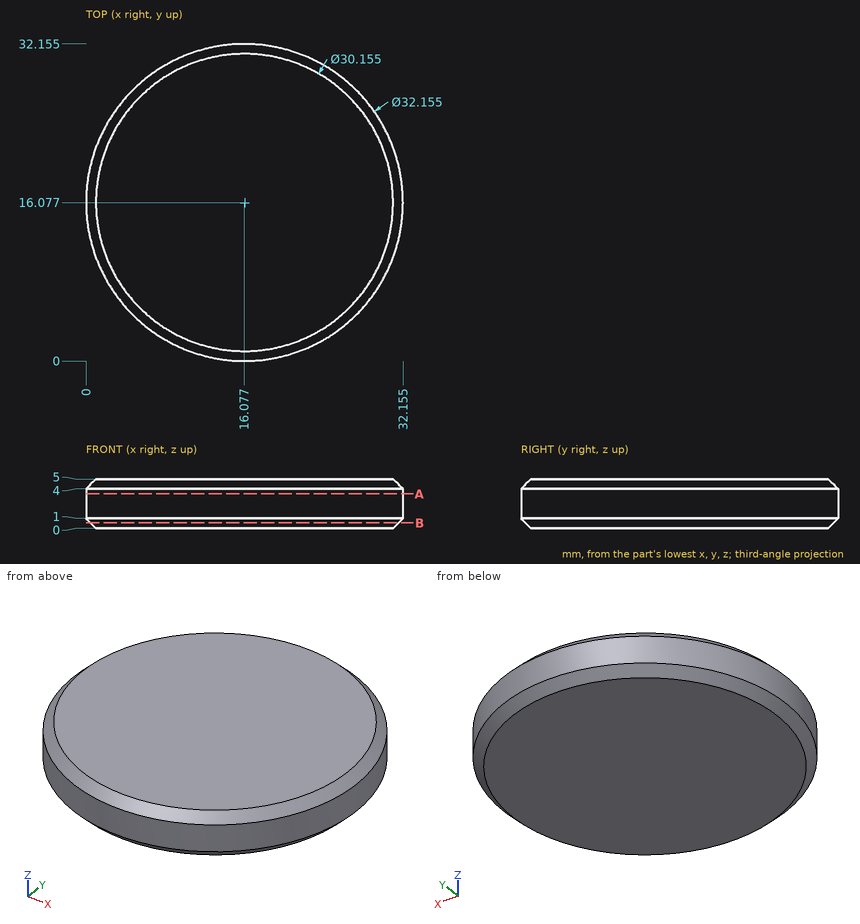
Here's the drawing with two shaded views (mm, measured from the low corner). I have some questions. Give positions to 0.01 mm unless a question says otherwise; leave off trailing zeros. Order: outer loops, then holes, each group sorted by start corner. A loop starts at its lowest first (then second) coordinate and runs counter-clockwise, first axis right, second up. Notation, with made-up numbers: (64.5, 19) -> (103.5, 19) arc R38 cw to (103.5, 57) -> close; hole circle Ø6 at (-6, 74.5). An arc over 180 degrees is marked (long way). One line per item, written item: value. Start each with the question number.
1. Imagine slicing it at A-A, the plane z = 3.5. List the corners of the cut face in (x, y) for me (1 decimal), plus the area to 3 significant figures.
2. I need wall thicknesses on probe 1 along X at (y, z) = (16, 2.7) (1 decimal); probe 2 along Y at (x, z) = (22.5, 1.5) (1 decimal); probe 3 along Y at (x, z) = (18, 4.3) (1 decimal). Which ranges of each line are inside material? Lowest first, please. Write a range as from..to.
3. Will this pin go through, and if not, where does the flat tip stop? pin 1 Ø4 at (x, y) = (20.5, 13) entering from -Z.
4. Imagine slicing it at B-B, the plane z = 0.55. List the corners of the cut face in (x, y) for me (1 decimal).
Values follow:
1. outline: circle Ø32.2 at (16.1, 16.1)
1. area: 812 mm2
2. probe 1: x = 0..32.2
2. probe 2: y = 1.3..30.8
2. probe 3: y = 0.4..31.7
3. pin 1: stops at z = 0
4. outline: circle Ø31.3 at (16.1, 16.1)
